```python
from build123d import *

# Parameters (mm, degrees)
SKETCH1_W           = 50
SKETCH1_H           = 110
BOSS_EXTRUDE1_DEPTH = 10
SKETCH2_W           = 12
SKETCH2_H           = 110
BOSS_EXTRUDE2_DEPTH = 120
SKETCH3_W           = 7.539466006
SKETCH3_H           = 40
BOSS_EXTRUDE3_DEPTH = 150


with BuildPart() as part:
    # Sketch1 → Boss-Extrude1 (new body)
    with BuildSketch(Plane.XY):
        with Locations((-25, 55)):
            Rectangle(SKETCH1_W, SKETCH1_H)
    extrude(amount=BOSS_EXTRUDE1_DEPTH)

    # Sketch2 → Boss-Extrude2 (add)
    with BuildSketch(Plane(origin=(0, 0, 0), x_dir=(-1, 0, 0), z_dir=(0, 0, -1))):
        with Locations((6, 55)):
            Rectangle(SKETCH2_W, SKETCH2_H)
    extrude(amount=BOSS_EXTRUDE2_DEPTH)

    # Sketch3 → Boss-Extrude3 (add)
    with BuildSketch(Plane.ZY.offset(12)):
        with Locations((-116.230266997, 55)):
            Rectangle(SKETCH3_W, SKETCH3_H)
    extrude(amount=BOSS_EXTRUDE3_DEPTH)


solid = part.part
```
The model under review builds one solid part; all positions refer to its coordinate system, in mm. A direction names the side the tool comes from. Give positions to 0.01 mm unless a question says otherwise; leave off trailing zeros. Write each loop counter-clockwise with the first axis right and the second up, starting at its lowest first coordinate (ties: lowest second). Pieces come first, ordered by that corner, then holes. Notation, with made-up numbers: (65, 18.25) -> (101, 18.25) arc R23 ccw to (101, 46.25) -> close; hole circle Ø11 at (23, 35.5). An arc over 180 degrees is marked (long way). Answer in a Markdown table with one row per item.
1) Clearance check with flat-ended pins moving along their axes: P1, Ø3, axis at y = 58, z = 4, coming from the -X side; P2, Ø6, axis at x = -78.5, z = -116.5, coming from the -Y side; P3, Ø20, axis at x = -120, y = 49, coming from the +Z side. State where each tip first meets the part, or that it passes through.
Worked answers:
| item | result |
|---|---|
| P1 | x = -50 |
| P2 | y = 35 |
| P3 | z = -112.46 |
2) Add section C-C on z = -25. State the section outline as (x, y) points, plus the area to 3 significant figures.
Worked answers:
| item | result |
|---|---|
| outline | (-12, 0) -> (0, 0) -> (0, 110) -> (-12, 110) -> close |
| area | 1,320 mm² |
3) Add section D-D on x = -109.5. State the section outline as (y, z) points, plus the area to 3 significant figures.
Worked answers:
| item | result |
|---|---|
| outline | (35, -120) -> (75, -120) -> (75, -112.46) -> (35, -112.46) -> close |
| area | 302 mm² |
4) Tool access review of faces 4 (the flat face through (-50, 54, 5)), 5 (the flat face through (-86, 75, -116)), 6 (the flat face through (-86, 35, -116)): name each direction out of +Z, -Z, +X, -X, +Y, -Y from which nothing blocks a thin tool from reaching the whole face with its end or side.
Worked answers:
| item | result |
|---|---|
| face 4 | +Z, -X, +Y, -Y |
| face 5 | -Z, -X, +Y |
| face 6 | -Z, -X, -Y |
5) For L1, parallel to Z at x = -33.5, y = 42; L2, parallel to Z at x = -129.5, y = 71.5; L3, parallel to X at y = 18, z = -88, list the stretches that pass through material, from the lowest coordinate up. Write a range as [from, to].
Worked answers:
| item | result |
|---|---|
| L1 | [-120, -112.46], [0, 10] |
| L2 | [-120, -112.46] |
| L3 | [-12, 0] |
6) Add section A-A on x = -39. State the section outline as (y, z) points.
Worked answers:
| item | result |
|---|---|
| outline | (0, 0) -> (110, 0) -> (110, 10) -> (0, 10) -> close; (35, -120) -> (75, -120) -> (75, -112.46) -> (35, -112.46) -> close |
7) Mouldability with a two-part tool opening along Z and no side actions: class faces 1 (the flat face through (-162, 55, -116)), 2 (the flat face through (-25, 56, 10)), 3 (the flat face through (-31, 56, 0)) as +Z half, -Z half, draft (parallel to the pull), parting line (faces both ways), or undercut.
Worked answers:
| item | result |
|---|---|
| face 1 | draft |
| face 2 | +Z half |
| face 3 | undercut |
8) Add section B-B on y = 82. State the section outline as (x, z) points.
Worked answers:
| item | result |
|---|---|
| outline | (-50, 0) -> (-12, 0) -> (-12, -120) -> (0, -120) -> (0, 10) -> (-50, 10) -> close |
